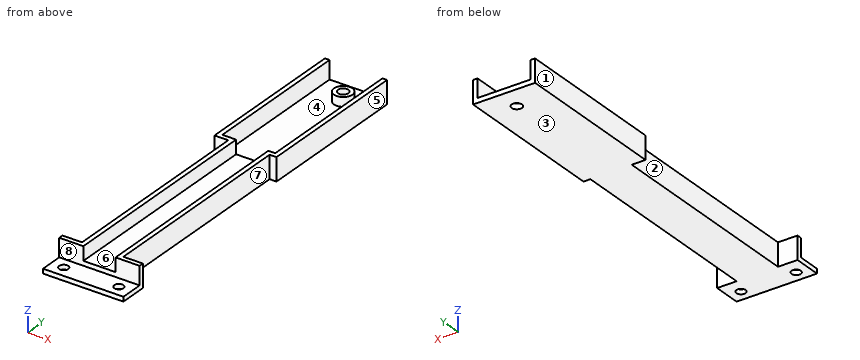
Autodesk Fusion 360 part; units mm, degrees
sketch "スケッチ1" plane through (0, 0, 0) normal (0, 0, 1) x (1, 0, 0)
  line L0 (-17.5, 170) -> (17.5, 170)
  line L1 (17.5, 170) -> (17.5, 0)
  line L2 (17.5, 0) -> (-17.5, 0)
  line L3 (-17.5, 0) -> (-17.5, 170)
  circle A0 centre (12, 5) radius 2
  circle A1 centre (-12, 5) radius 2
  line L4 (12, 5) -> (-12, 5) construction
  circle A2 centre (0, 160) radius 2.25
  dimension "d1" = 170
  dimension "d2" = 35
  dimension "d3" = 4
  dimension "d4" = 4
  dimension "d5" = 24
  dimension "d6" = 5
  dimension "d7" = 5.5
  dimension "d8" = 4.5
  dimension "d9" = 155
extrude "押し出し1" add sketch "スケッチ1" along normal blind 2 makes body 1
sketch "スケッチ2" plane through (0, 0, 2) normal (0, 0, 1) x (-1, 0, 0)
  circle A0 centre (-12, -5) radius 2
  circle A1 centre (0, -160) radius 2.25
  circle A2 centre (12, -5) radius 2
  line L0 (17.5, 0) -> (-17.5, 0)
  line L1 (-17.5, 0) -> (-17.5, -170)
  line L2 (-17.5, -170) -> (17.5, -170)
  line L3 (17.5, -170) -> (17.5, 0)
  line L4 (-7, -170) -> (-17.5, -170)
  line L5 (-17.5, -170) -> (-17.5, -10)
  line L6 (-17.5, -10) -> (-7, -10)
  line L7 (-7, -10) -> (-7, -170)
  line L8 (17.5, -170) -> (7, -170)
  line L9 (7, -170) -> (7, -10)
  line L10 (7, -10) -> (17.5, -10)
  line L11 (17.5, -10) -> (17.5, -170)
  dimension "d12" = 10.5
  dimension "d13" = 10
  dimension "d14" = 10.5
  dimension "d15" = 10
extrude "押し出し2" cut sketch "スケッチ2" against normal blind 2 contours L2 L3 L8 L9 L10 L11 | L1 L2 L4 L5 L6 L7 bodies 1
sketch "スケッチ3" plane through (7, 0, 0) normal (1, 0, 0) x (0, 1, 0)
  line L0 (170, 2) -> (10, 2)
  line L1 (10, 2) -> (10, 0)
  line L2 (10, 0) -> (170, 0)
  line L3 (170, 0) -> (170, 2)
  line L4 (10, 10) -> (104, 10)
  line L5 (104, 10) -> (104, 0)
  line L6 (104, 0) -> (10, 0)
  line L7 (10, 0) -> (10, 10)
  dimension "d18" = 10
  dimension "d19" = 94
extrude "押し出し3" add sketch "スケッチ3" along normal blind 2 separate body contours L0 L1 L2 L5 L6 L7 | L0 L4 L5 L7 makes body 2
sketch "スケッチ4" plane through (-7, 0, 0) normal (-1, 0, 0) x (0, -1, 0)
  line L0 (-10, 2) -> (-170, 2)
  line L1 (-170, 2) -> (-170, 0)
  line L2 (-170, 0) -> (-10, 0)
  line L3 (-10, 0) -> (-10, 2)
  line L4 (-10, 10) -> (-104, 10)
  line L5 (-104, 10) -> (-104, 0)
  line L6 (-104, 0) -> (-10, 0)
  line L7 (-10, 0) -> (-10, 10)
  line L8 (-104, 10) -> (-104, 0)
  line L9 (-10, 0) -> (-10, 10)
  line L10 (-10, 10) -> (-104, 10)
extrude "押し出し4" add sketch "スケッチ4" along normal blind 2 separate body contours L0 L2 L3 L5 L6 L7 L8 L9 | L0 L4 L5 L7 L8 L9 L10 makes body 3
sketch "スケッチ5" plane through (0, 0, 2) normal (0, 0, 1) x (-1, 0, 0)
  line L0 (7, -170) -> (7, -10)
  line L1 (7, -10) -> (17.5, -10)
  line L2 (17.5, -10) -> (17.5, 0)
  line L3 (17.5, 0) -> (-17.5, 0)
  line L4 (-17.5, 0) -> (-17.5, -10)
  line L5 (-17.5, -10) -> (-7, -10)
  line L6 (-7, -10) -> (-7, -170)
  line L7 (-7, -170) -> (7, -170)
  circle A0 centre (12, -5) radius 2
  circle A1 centre (0, -160) radius 2.25
  circle A2 centre (-12, -5) radius 2
  line L8 (-7, -170) -> (-10, -170)
  line L9 (-10, -170) -> (-10, -104)
  line L10 (-10, -104) -> (-7, -104)
  line L11 (-7, -104) -> (-7, -170)
  line L12 (-7, -104) -> (-9, -104)
  line L13 (7, -170) -> (13, -170)
  line L14 (13, -170) -> (13, -104)
  line L15 (13, -104) -> (7, -104)
  line L16 (7, -104) -> (7, -170)
  line L17 (7, -104) -> (9, -104)
  dimension "d24" = 3
  dimension "d25" = 6
extrude "押し出し5" add sketch "スケッチ5" against normal blind 2 contours L0 L13 L14 L15 L16 L17 | L6 L8 L9 L10 L11 L12 bodies 1 2 3
sketch "スケッチ10" plane through (-13, 0, 0) normal (-1, 0, 0) x (0, -1, 0)
  line L0 (-104, 2) -> (-170, 2)
  line L1 (-170, 2) -> (-170, 0)
  line L2 (-170, 0) -> (-104, 0)
  line L3 (-104, 0) -> (-104, 2)
  line L4 (-104, 0) -> (-170, 0)
  line L5 (-170, 0) -> (-170, 10)
  line L6 (-170, 10) -> (-104, 10)
  line L7 (-104, 10) -> (-104, 0)
  point P0 (-104, 10)
extrude "押し出し8" add sketch "スケッチ10" along normal blind 2 separate body makes body 4
sketch "スケッチ11" plane through (10, 0, 0) normal (1, 0, 0) x (0, 1, 0)
  line L0 (170, 2) -> (104, 2)
  line L1 (104, 2) -> (104, 0)
  line L2 (104, 0) -> (170, 0)
  line L3 (170, 0) -> (170, 2)
  line L4 (104, 0) -> (170, 0)
  line L5 (170, 0) -> (170, 10)
  line L6 (170, 10) -> (104, 10)
  line L7 (104, 10) -> (104, 0)
  line L8 (104, 10) -> (10, 10)
extrude "押し出し9" add sketch "スケッチ11" along normal blind 2 separate body makes body 5
sketch "スケッチ12" plane through (0, 104, 0) normal (0, -1, 0) x (1, 0, 0)
  line L0 (-13, 0) -> (-13, 10)
  line L1 (-13, 10) -> (-15, 10)
  line L2 (-15, 10) -> (-15, 0)
  line L3 (-15, 0) -> (-13, 0)
  line L4 (-15, 10) -> (-7, 10)
  line L5 (-7, 10) -> (-7, 0)
  line L6 (-7, 0) -> (-15, 0)
  line L7 (-15, 0) -> (-15, 10)
  line L8 (-7, 2) -> (-7, 10)
  line L9 (17.5, 0) -> (-17.5, 0)
  line L10 (7, 10) -> (12, 10)
  line L11 (12, 10) -> (12, 0)
  line L12 (12, 0) -> (7, 0)
  line L13 (7, 0) -> (7, 10)
  line L14 (12, 10) -> (12, 0)
  line L15 (7, 2) -> (7, 10)
  line L16 (10, 10) -> (12, 10)
extrude "押し出し10" add sketch "スケッチ12" along normal blind 2 bodies 1 4 5
sketch "スケッチ13" plane through (0, 10, 0) normal (0, 1, 0) x (-1, 0, 0)
  line L0 (-9, 0) -> (-9, 2)
  line L1 (-9, 2) -> (-17.5, 2)
  line L2 (-17.5, 2) -> (-17.5, 0)
  line L3 (-17.5, 0) -> (-9, 0)
  line L4 (-17.5, 0) -> (-7, 0)
  line L5 (-7, 0) -> (-7, 10)
  line L6 (-7, 10) -> (-17.5, 10)
  line L7 (-17.5, 10) -> (-17.5, 0)
  line L8 (7, 10) -> (17.5, 10)
  line L9 (17.5, 10) -> (17.5, 0)
  line L10 (17.5, 0) -> (7, 0)
  line L11 (7, 0) -> (7, 10)
  point P0 (-7, 10)
  point P1 (7, 10)
  point P2 (17.5, 0)
extrude "押し出し11" add sketch "スケッチ13" along normal blind 2 bodies 1
sketch "スケッチ14" plane through (0, 0, 2) normal (0, 0, 1) x (-1, 0, 0)
  line L0 (7, -104) -> (7, -10)
  line L1 (7, -10) -> (17.5, -10)
  line L2 (17.5, -10) -> (17.5, 0)
  line L3 (17.5, 0) -> (-17.5, 0)
  line L4 (-17.5, 0) -> (-17.5, -10)
  line L5 (-17.5, -10) -> (-7, -10)
  line L6 (-7, -10) -> (-7, -104)
  line L7 (-7, -104) -> (-10, -104)
  line L8 (-10, -104) -> (-10, -170)
  line L9 (-10, -170) -> (13, -170)
  line L10 (13, -170) -> (13, -104)
  line L11 (13, -104) -> (7, -104)
  circle A0 centre (12, -5) radius 2
  circle A1 centre (0, -160) radius 2.25
  circle A2 centre (-12, -5) radius 2
  line L12 (7, -104) -> (-7, -104)
  line L13 (-7, -104) -> (-7, -10)
  line L14 (-7, -10) -> (7, -10)
  line L15 (7, -10) -> (7, -104)
extrude "押し出し12" add sketch "スケッチ14" along normal blind 2 contours L0 L6 L12 L13 L14 L15 bodies 1
sketch "スケッチ15" plane through (0, 0, 2) normal (0, 0, 1) x (-1, 0, 0)
  circle A0 centre (0, -160) radius 2.25
  line L0 (13, -104) -> (-10, -104)
  line L1 (-10, -104) -> (-10, -170)
  line L2 (-10, -170) -> (13, -170)
  line L3 (13, -170) -> (13, -104)
  circle A1 centre (0, -160) radius 4
  dimension "d43" = 8
extrude "押し出し13" add sketch "スケッチ15" along normal blind 4 contours A1 bodies 1
Input: part model. Units: mm. Frame: model coordinates. Face numbers are marked on the shaded views. A direction names the side the tool comes from. Coordinates: 2 decimals unless noted, no trailing zeros. Loops run counter-clockwise (first coordinate to the right, second up) from the corner with the lowest first, then second, coordinate; pieces in that order, holes last.
Q1. Mould query, pull axis Y, two halves, no side actions, for the marked faces 6, 7 and 8. Classes: +Y half, -Y half, draft (parallel to the pull), parting line (faces both ways), or undercut.
Results are:
face 6: draft
face 7: undercut
face 8: -Y half
Q2. Section C-C, the plane y = 5. Return the cut outline in (x, z), and give its area (3 significant figures).
Results are:
outline: (-17.5, 0) - (-14, 0) - (-14, 2) - (-17.5, 2) - close; (-10, 0) - (10, 0) - (10, 2) - (-10, 2) - close; (14, 0) - (17.5, 0) - (17.5, 2) - (14, 2) - close
area: 54.0 mm2
Q3. Section D-D, the plane x = 15.5. Return the cut outline in (y, z).
Results are:
outline: (0, 0) - (12, 0) - (12, 10) - (10, 10) - (10, 2) - (0, 2) - close
Q4. Section B-B, the plane y = 160. Return the cut outline in (x, z), and give its area (3 significant figures).
Results are:
outline: (-15, 0) - (-2.25, 0) - (-2.25, 6) - (-4, 6) - (-4, 2) - (-13, 2) - (-13, 10) - (-15, 10) - close; (2.25, 0) - (12, 0) - (12, 10) - (10, 10) - (10, 2) - (4, 2) - (4, 6) - (2.25, 6) - close
area: 91.0 mm2
Q5. Line query: line 1 along X through (y, z) = (160, 4.3); line 2 along Y through (x, z) = (0, 2.9); line 3 along Y through (x, z) = (-12, 1.55). Output: solid intervals per line, ascending.
Results are:
line 1: x = -15 to -13, -4 to -2.25, 2.25 to 4, 10 to 12
line 2: y = 10 to 104, 156 to 157.75, 162.25 to 164
line 3: y = 0 to 3, 7 to 12, 102 to 170
Q6. Set-up query: the marked faces 1, 2, 3, 4 and 5. Return all of +Z, -Z, +X, -X, +Y, -Y with unobstructed straight access to the full face (end or side cutting, diameter ignored); none if empty.
Results are:
face 1: +Z, -Z, -X, +Y
face 2: +Z, -Z, -X
face 3: -Z, +X, -X, +Y, -Y
face 4: +Z
face 5: +Z, -Z, +X, +Y
Q7. Contact query for flat-ended pins moving along their axis: pin 1 (4 mm diameter, centred on y = 104, z = 1.5, fed in from -X); pin 2 (1.5 mm diameter, centred on x = -2, y = 126, fed in from +Z); pin 3 (5 mm diameter, centred on y = 54, z = 8.5, fed in from -X); pin 4 (12 mm diameter, centred on x = 3.5, y = 100, fed in from +Z). Output: stop coordinate, or through.
Results are:
pin 1: stops at x = -15
pin 2: stops at z = 2
pin 3: stops at x = -9
pin 4: stops at z = 10
Q8. Section A-A, the plane z = 8.5. Return the cut outline in (x, y), and give its area (3 significant figures).
Results are:
outline: (-17.5, 10) - (-7, 10) - (-7, 104) - (-13, 104) - (-13, 170) - (-15, 170) - (-15, 102) - (-9, 102) - (-9, 12) - (-17.5, 12) - close; (7, 10) - (17.5, 10) - (17.5, 12) - (9, 12) - (9, 102) - (12, 102) - (12, 170) - (10, 170) - (10, 104) - (7, 104) - close
area: 692 mm2
